Read the model definition and answer for the solid it produces. Units are mm, in the model's axes. Coordinates: 2 decimals unless noted, no trailing zeros. Loops run counter-clockwise (first coordinate to the right, second up) from the corner with the lowest first, then second, coordinate; pieces in that order, holes last.
from build123d import *

# Parameters (mm, degrees)
F0_W     = 62
F0_H     = 62
F1_DEPTH = 3
F2_R     = 3.5
F2_R_2   = 12.75
F3_DEPTH = 25
F4_R     = 3


with BuildPart() as f1:
    # F0 (on Top) → F1 (new body)
    with BuildSketch(Plane.XY):
        Rectangle(F0_W, F0_H)
    extrude(amount=F1_DEPTH)

    # F2 (on face) → F3 (cut)
    with BuildSketch(Plane.XY.offset(3)):
        with Locations((-20, 20)):
            Circle(F2_R)
        with Locations((20, 20)):
            Circle(F2_R)
        with Locations((20, -20)):
            Circle(F2_R)
        with Locations((-20, -20)):
            Circle(F2_R)
        Circle(F2_R_2)
    extrude(amount=-F3_DEPTH, mode=Mode.SUBTRACT)

    # F4
    f4_edges = [f1.edges().sort_by_distance(p)[0] for p in [
        (-31, 31, 1.5),
        (31, 31, 1.5),
        (-31, -31, 1.5),
        (31, -31, 1.5),
    ]]
    fillet(f4_edges, radius=F4_R)


solid = f1.part
Q1. Determine the mould class of faces 1 (the face through (-18.12, 22.95, 1.52)), 2 (the face through (-30.14, -30.1, 1.52)), 3 (the face through (-14, 0, 3)) for opening direction X: +X half, -X half, draft (parallel to the pull), parting line (faces both ways), or undercut.
Findings below:
face 1: undercut
face 2: -X half
face 3: draft
Q2. A cutting plane is placed at D-D (z = 2.35). Give the vertices of the cut face in (x, y).
Findings below:
outline: (-31, -28) arc R3 ccw to (-28, -31) - (28, -31) arc R3 ccw to (31, -28) - (31, 28) arc R3 ccw to (28, 31) - (-28, 31) arc R3 ccw to (-31, 28) - close; hole circle Ø7 at (-20, -20); hole circle Ø7 at (-20, 20); hole circle Ø25.5 at (0, 0); hole circle Ø7 at (20, -20); hole circle Ø7 at (20, 20)
Q3. A cutting plane is placed at A-A (x = -20). Give the vertices of the cut face in (y, z), then the cut area to 3 significant figures.
Findings below:
outline: (-31, 0) - (-23.5, 0) - (-23.5, 3) - (-31, 3) - close; (-16.5, 0) - (16.5, 0) - (16.5, 3) - (-16.5, 3) - close; (23.5, 0) - (31, 0) - (31, 3) - (23.5, 3) - close
area: 144 mm2
Q4. Flat-ended cylindrical pins translate along their axes: pin 1 Ø5 at (x, y) = (-17, 21) entering from -Z; pin 2 Ø4 at (x, y) = (20, -20) entering from +Z. Find the tip coordinate at first contact, or state that the pin passes through.
Findings below:
pin 1: stops at z = 0
pin 2: passes through
Q5. A cutting plane is placed at C-C (x = 0). Give the vertices of the cut face in (y, z).
Findings below:
outline: (-31, 0) - (-12.75, 0) - (-12.75, 3) - (-31, 3) - close; (12.75, 0) - (31, 0) - (31, 3) - (12.75, 3) - close
Q6. Straight lines are drawn through the part: probe 1 along Y at (x, z) = (20, 1.9); probe 2 along Y at (x, z) = (0, 2.4); probe 3 along Y at (x, z) = (17, 1.55). For each, find the intervals that lie inside material, in ascending order.
Findings below:
probe 1: y = -31 to -23.5, -16.5 to 16.5, 23.5 to 31
probe 2: y = -31 to -12.75, 12.75 to 31
probe 3: y = -31 to -21.8, -18.2 to 18.2, 21.8 to 31
